Check sheet for the drawn part. Datum: minimum x, y, z corner. Units: mm. A direction names the side the tool comes from. Round coordinates to 2 decimals unless told otherwise and drop trailing zeros. Order: outer loops, then holes, each group sorted by start corner. A loop starts at its lowest first (then second) coordinate and runs counter-clockwise, first axis right, second up. Notation, with made-up numbers: M 84,87.5 L 99,87.5 A30 ccw 99,118.5 Z; hole C 49,7 d8. An arc over 180 degrees is marked long. Use one line per item in the form item = value. Start each with the question number.
Item 1: Go/stop test with flat-tipped pins: pin 1 Ø0.6 at (y, z) = (54.5, 27.5) entering from +X; pin 2 Ø1.6 at (y, z) = (1, 27.5) entering from -X; pin 3 Ø0.6 at (x, z) = (25.5, 27) entering from -Y. Record where each tip stops, or that it passes through.
Item 2: Cross-section at A-A on y = 95.5. Enter the section's corners in (x, z).
Item 3: Cross-section at C-C on y = 72. Enter the section's corners in (x, z).
Item 4: Tool access check on the marked faces 1 and 2. Record the directions out of +Z, -Z, +X, -X, +Y, -Y that give a thin tool (end or side, any length) a straight path to the whole face; none if there is none.
Item 5: Cross-section at B-B on x = 20.5. Enter the section's corners in (y, z), then the cut area to 3 significant figures.
Item 6: Cross-section at D-D on x = 13.5. Enter the section's corners in (y, z).
Item 7: Thickness scan on probe 1 along Y at (x, z) = (0.7, 7.5); probe 2 along X at (y, z) = (69.5, 25); probe 3 along Z at (x, y) = (13.5, 14). Record the ranges inside material, lowest first. Write a range as [from, to].
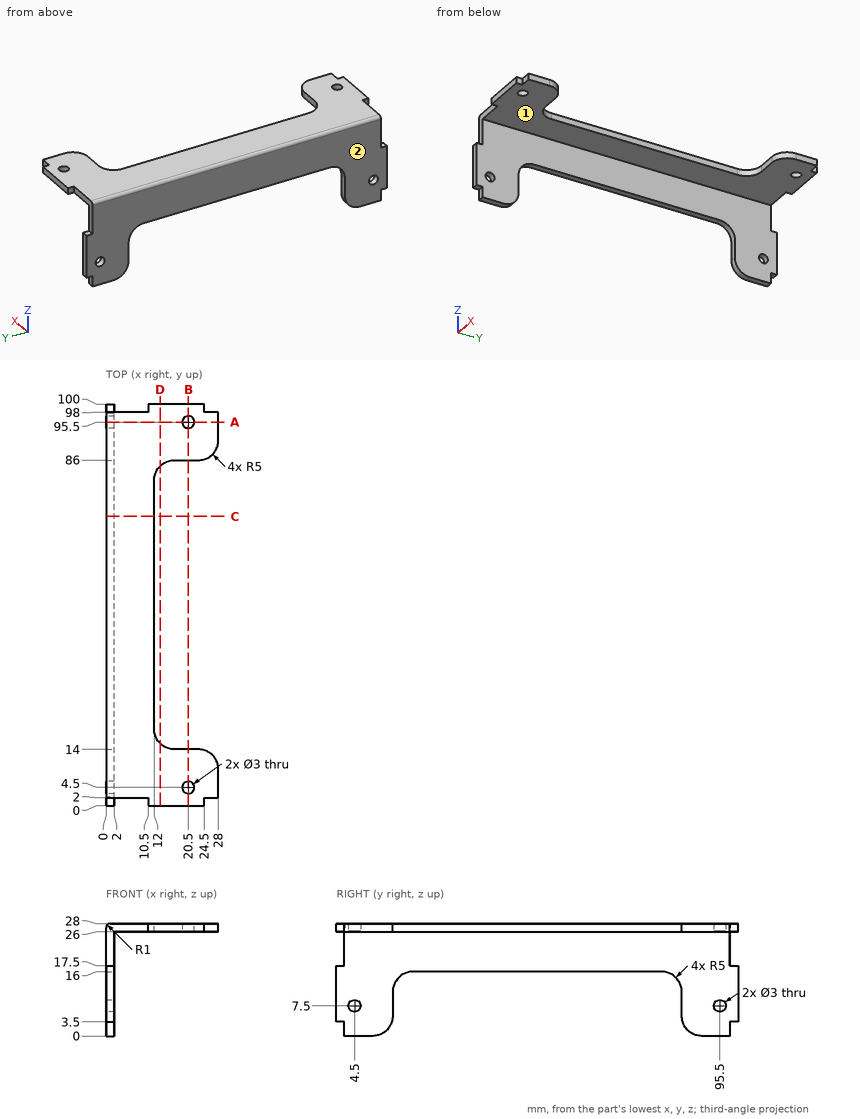
Output values:
q1.pin_1 = 12
q1.pin_2 = 10.5
q1.pin_3 = 2
q2.outline = M 0,0 L 2,0 L 2,6 L 0,6 Z; M 0,9 L 2,9 L 2,26 L 19,26 L 19,28 L 1,28 A1 ccw 0,27 Z; M 22,26 L 28,26 L 28,28 L 22,28 Z
q3.outline = M 0,16 L 2,16 L 2,26 L 12,26 L 12,28 L 1,28 A1 ccw 0,27 Z
q4.face_1 = -Z, +X, +Y, -Y
q4.face_2 = +Z, -Z, -X, +Y, -Y
q5.outline = M 0,26 L 3,26 L 3,28 L 0,28 Z; M 6,26 L 14,26 L 14,28 L 6,28 Z; M 86,26 L 94,26 L 94,28 L 86,28 Z; M 97,26 L 100,26 L 100,28 L 97,28 Z
q5.area = 44.0 mm2
q6.outline = M 0,26 L 15.43,26 L 15.43,28 L 0,28 Z; M 84.57,26 L 100,26 L 100,28 L 84.57,28 Z
q7.probe_1 = [0, 3], [6, 14], [86, 94], [97, 100]
q7.probe_2 = [0, 2]
q7.probe_3 = [26, 28]
